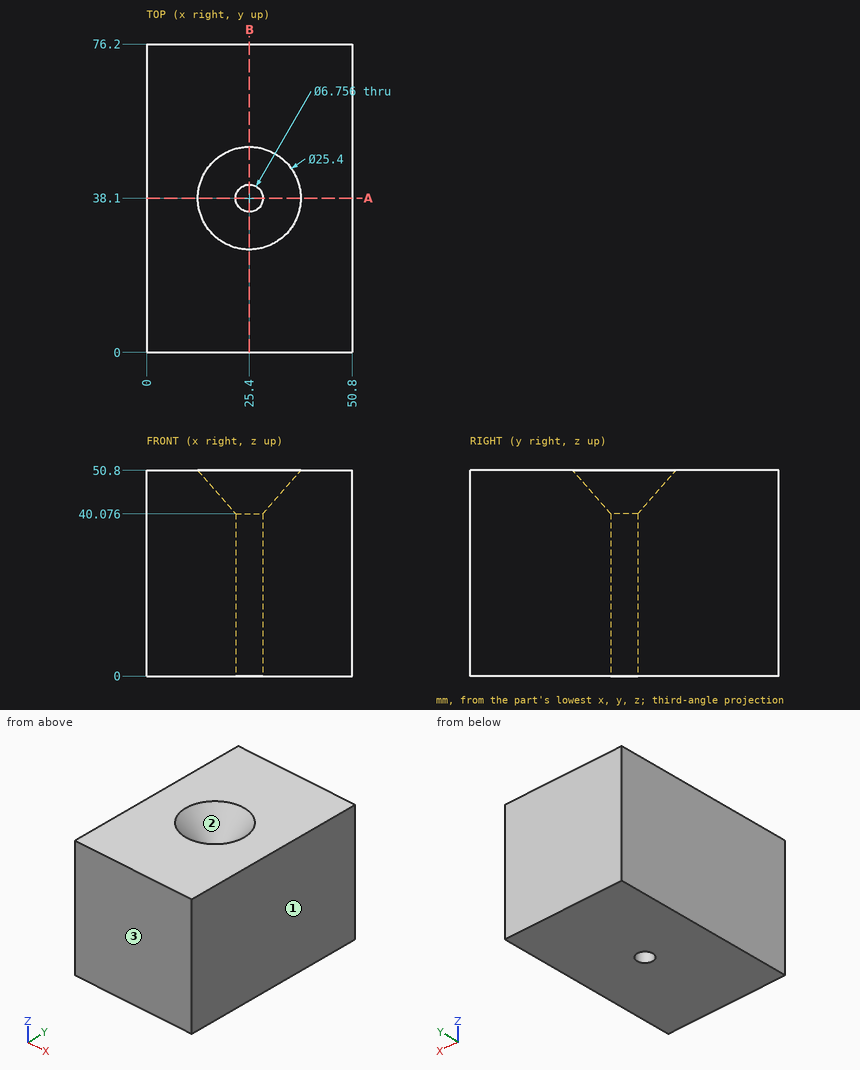
Geometry check sheet. Reference: drawing and pictorial views, mm from the part's lowest x, y, z. Coordinates: 2 decimals unless noted, no trailing zeros. Order: outer loops, then holes, each group sorted by start corner. A loop starts at its lowest first (then second) coordinate and runs counter-clockwise, first axis right, second up.
1. Go/stop test with a flat-tipped pin: pin 1 Ø9 at (x, y) = (25.4, 38.1) entering from +Z (1 decimal). Record where the tip stops, or that it passes through.
Results found:
pin 1: stops at z = 41.4
2. Release check for a two-part mould opening along Y. For the marked faces 1, 2 and 3 record: +Y half, -Y half, draft (parallel to the pull), parting line (faces both ways), or undercut.
Results found:
face 1: draft
face 2: undercut
face 3: -Y half
3. Sectioned sample at A-A, the plane y = 38.1. Record the cut outline in (x, z).
Results found:
outline: (0, 0) - (22.02, 0) - (22.02, 40.08) - (12.7, 50.8) - (0, 50.8) - close; (28.78, 0) - (50.8, 0) - (50.8, 50.8) - (38.1, 50.8) - (28.78, 40.08) - close
4. Scan lines: line 1 (X direction, y = 38, z = 30); line 2 (Y direction, x = 25.4, z = 24.5); line 3 (X direction, y = 37, z = 29) (1 decimal). Record each from-to range of solid material in increasing order.
Results found:
line 1: x = 0 to 22.02, 28.78 to 50.8
line 2: y = 0 to 34.72, 41.48 to 76.2
line 3: x = 0 to 22.2, 28.6 to 50.8
5. Sectioned sample at B-B, the plane x = 25.4. Record the cut outline in (y, z), and give its area (3 significant figures).
Results found:
outline: (0, 0) - (34.72, 0) - (34.72, 40.08) - (25.4, 50.8) - (0, 50.8) - close; (41.48, 0) - (76.2, 0) - (76.2, 50.8) - (50.8, 50.8) - (41.48, 40.08) - close
area: 3,430 mm2
